```python
from build123d import *

# Parameters (mm, degrees)
SKETCH1_W           = 92
SKETCH1_H           = 150
BOSS_EXTRUDE1_DEPTH = 8
SKETCH2_W           = 30
SKETCH2_H           = 8
SKETCH2_W_2         = 8
SKETCH2_H_2         = 30
BOSS_EXTRUDE2_DEPTH = 8
CUT_EXTRUDE2_DEPTH  = 9


with BuildPart() as part:
    # Sketch1 → Boss-Extrude1 (new body)
    with BuildSketch(Plane(origin=(0, 0, 0), x_dir=(0, 0, -1), z_dir=(1, 0, 0))):
        with Locations((46, 75)):
            Rectangle(SKETCH1_W, SKETCH1_H)
    extrude(amount=BOSS_EXTRUDE1_DEPTH)

    # Sketch2 → Boss-Extrude2 (add)
    with BuildSketch(Plane.ZY):
        with Locations((-46, 154)):
            Rectangle(SKETCH2_W, SKETCH2_H)
        with Locations((-46, -4)):
            Rectangle(SKETCH2_W, SKETCH2_H)
        with Locations((4, 40)):
            Rectangle(SKETCH2_W_2, SKETCH2_H_2)
        with Locations((4, 110)):
            Rectangle(SKETCH2_W_2, SKETCH2_H_2)
        with Locations((-96, 40)):
            Rectangle(SKETCH2_W_2, SKETCH2_H_2)
        with Locations((-96, 110)):
            Rectangle(SKETCH2_W_2, SKETCH2_H_2)
    extrude(amount=-BOSS_EXTRUDE2_DEPTH)

    # Sketch4 → Cut-Extrude2 (cut, through all)
    with BuildSketch(Plane(origin=(8, 0, 0), x_dir=(0, 0, -1), z_dir=(1, 0, 0))):
        with BuildLine():
            Line((97, 85), (97, 65))
            ThreePointArc((97, 65), (92, 60), (87, 65))
            Line((87, 65), (87, 85))
            ThreePointArc((87, 85), (92, 90), (97, 85))
        make_face()
        Polygon((0, 76.65), (4, 76.65), (4, 78.5), (6.2, 78.5), (6.2, 76.65), (8.5, 76.65), (8.5, 73.35), (6.2, 73.35), (6.2, 71.5), (4, 71.5), (4, 73.35), (0, 73.35), align=None)
        Polygon((78.15, 0), (78.15, 4), (80, 4), (80, 6.2), (78.15, 6.2), (78.15, 8.5), (74.85, 8.5), (74.85, 6.2), (73, 6.2), (73, 4), (74.85, 4), (74.85, 0), align=None)
        Polygon((74.85, 150), (78.15, 150), (78.15, 146), (80, 146), (80, 143.8), (78.15, 143.8), (78.15, 141.5), (74.85, 141.5), (74.85, 143.8), (73, 143.8), (73, 146), (74.85, 146), align=None)
    extrude(amount=-CUT_EXTRUDE2_DEPTH, mode=Mode.SUBTRACT)


solid = part.part
```
Geometry: final body of the model. Coordinates: model frame, mm. A direction names the side the tool comes from. Round coordinates to 2 decimals unless told otherwise and drop trailing zeros. Loops run counter-clockwise (first coordinate to the right, second up) from the corner with the lowest first, then second, coordinate; pieces in that order, holes last. Notation, with made-up numbers: (36.5, 77.25) -> (51.5, 77.25) arc R34 cw to (51.5, 115.25) -> close; hole circle Ø7 at (68.25, 37). An arc over 180 degrees is marked (long way). Use one line per item in the form item = value. Start each with the question number.
1) Section B-B on z = -69.5. Output: boundary loops of the cut face in (x, y).
2) First-contact query: P1, Ø1.2, axis at x = 5, y = 142, coming from the -Z side; P2, Ø1.5, axis at x = 5.5, y = 78, coming from the -Z side; P3, Ø4, axis at x = 6, z = -76.5, coming from the -Y side. Flat tips, straight axial feed; report the tip coordinate or a pass-through.
3) Line query: L1, parallel to Z at x = 6, y = 72; L2, parallel to Y at x = 4.75, z = -21.5; L3, parallel to Z at x = 2, y = 79. Output: solid intervals per line, ascending.
4) Section A-A on y = 131.5. Output: boundary loops of the cut face in (x, z).
5) Access query for faces 4 (the flat face through (4, 75, -8.5)), 5 (the flat face through (4, 25, -96)), 6 (the flat face through (4, 137, 0)), 7 (the flat face through (4, 148, -78.15)). Directions: +Z, -Z, +X, -X, +Y, -Y. A direction counts if a zero-diameter tool reaches every point of the face in a straight line with its end or side. Return the directions, or none.
6) Draft query along Z for faces 1 (the flat face through (4, 154, -61)), 2 (the flat face through (4, 2, -74.85)), 3 (the flat face through (4, 125, 4)). Return one class per face: released by +Z, released by -Z, zero draft, split by the parting line, or undercut.
Response:
q1.outline = (0, 0) -> (8, 0) -> (8, 150) -> (0, 150) -> close
q2.P1 = -92
q2.P2 = -87
q2.P3 = 0
q3.L1 = -87 to -6.2, -4 to 0
q3.L2 = 0 to 150
q3.L3 = -87 to 0
q4.outline = (0, -92) -> (8, -92) -> (8, 0) -> (0, 0) -> close
q5.face_4 = +Z, +X, -X
q5.face_5 = -Z, +X, -X, -Y
q5.face_6 = +Z, +X, -X, +Y
q5.face_7 = +X, -X, +Y
q6.face_1 = released by -Z
q6.face_2 = undercut
q6.face_3 = zero draft
